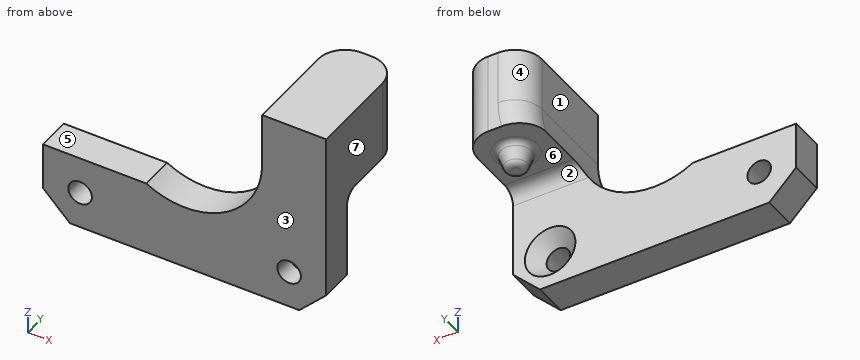
```python
from build123d import *

# Parameters (mm, degrees)
CROQUIS1_R              = 1.75
SALIENTE_EXTRUIR1_DEPTH = 5
CHAFL_N1_SIZE           = 2
SALIENTE_EXTRUIR2_DEPTH = 17.5
CROQUIS4_R              = 2.5
SALIENTE_EXTRUIR3_DEPTH = 3
NGULO_DE_SALIDA1_ANGLE  = 20
REDONDEO1_R             = 1
CHAFL_N2_SIZE           = 4
REDONDEO2_R             = 2
REDONDEO4_R             = 4


with BuildPart() as part:
    # Croquis1 → Saliente-Extruir1 (new body)
    with BuildSketch(Plane(origin=(0, 0, 0), x_dir=(1, 0, 0), z_dir=(0, 1, 0))):
        with BuildLine():
            Line((-21, 21), (21, 21))
            Line((21, 21), (21, -8))
            Line((21, -8), (11.5, -8))
            Line((11.5, -8), (11.5, 0))
            ThreePointArc((11.5, 0), (5.785436631, 9.938748562), (-5.678908346, 10))
            Line((-5.678908346, 10), (-21, 10))
            Line((-21, 10), (-21, 21))
        make_face()
        with Locations((-15.5, 15.5)):
            Circle(CROQUIS1_R, mode=Mode.SUBTRACT)
        with Locations((15.5, 15.5)):
            Circle(CROQUIS1_R, mode=Mode.SUBTRACT)
    extrude(amount=SALIENTE_EXTRUIR1_DEPTH)

    # Chaflán1
    chafl_n1_edges = [part.edges().sort_by_distance(p)[0] for p in [
        (13.75, 5, -15.5),
    ]]
    chamfer(chafl_n1_edges, length=CHAFL_N1_SIZE)

    # Croquis3 → Saliente-Extruir2 (add)
    with BuildSketch(Plane.XZ):
        with BuildLine():
            Line((10.781929326, -4), (21, -4))
            Line((21, -4), (21, 0))
            Line((21, 0), (21, 8))
            Line((21, 8), (11.5, 8))
            Line((11.5, 8), (11.5, 0))
            ThreePointArc((11.5, 0), (11.319058867, -2.031971056), (10.781929326, -4))
        make_face()
    extrude(amount=-SALIENTE_EXTRUIR2_DEPTH)

    # Croquis4 → Saliente-Extruir3 (add)
    with BuildSketch(Plane(origin=(0, 0, -4), x_dir=(-1, 0, 0), z_dir=(0, 0, -1))):
        with Locations((-16.25, 12)):
            Circle(CROQUIS4_R)
    extrude(amount=SALIENTE_EXTRUIR3_DEPTH)

    # Ángulo de salida1
    ngulo_de_salida1_faces = [part.faces().sort_by_distance(p)[0] for p in [
        (18.75, 12, -5.5),
    ]]
    draft(ngulo_de_salida1_faces, Plane(origin=(10.781929326, 17.5, -4), x_dir=(-1, 0, 0), z_dir=(0, 0, -1)), NGULO_DE_SALIDA1_ANGLE)

    # Redondeo1
    redondeo1_edges = [part.edges().sort_by_distance(p)[0] for p in [
        (18.75, 12, -4),
        (17.658089297, 12, -7),
    ]]
    fillet(redondeo1_edges, radius=REDONDEO1_R)

    # Chaflán2
    chafl_n2_edges = [part.edges().sort_by_distance(p)[0] for p in [
        (-21, 2.5, -21),
        (21, 2.5, -21),
    ]]
    chamfer(chafl_n2_edges, length=CHAFL_N2_SIZE)

    # Redondeo2
    redondeo2_edges = [part.edges().sort_by_distance(p)[0] for p in [
        (15.890964663, 5, -4),
    ]]
    fillet(redondeo2_edges, radius=REDONDEO2_R)

    # Redondeo4
    redondeo4_edges = [part.edges().sort_by_distance(p)[0] for p in [
        (21, 17.5, 2),
        (11.319058867, 17.5, -2.031971056),
        (11.5, 17.5, 4),
    ]]
    fillet(redondeo4_edges, radius=REDONDEO4_R)


solid = part.part
```
Can you work these out from the model? Positions are in its coordinate system, mm. Face numbers are marked on the shaded views. A direction names the side the tool comes from. Coordinates: 2 decimals unless noted, no trailing zeros. Loops run counter-clockwise (first coordinate to the right, second up) from the corner with the lowest first, then second, coordinate; pieces in that order, holes last. Notation, with made-up numbers: M 60,-5 L 118,-5 A27 cw 118,26 Z; hole C 81,58.25 d5. An arc over 180 degrees is marked long. Put each result on its own line as item: value. Start each with the question number.
(1) Which directions (+Z, -Z, +X, -X, +Y, -Y) give clear straight access to the entire face, cutting with the end or side of a thin tool? Please do the marked faces 4, 5, 6 and 7.
(2) Imagine slicing it at D-D on z = 5.5. List the corners of the cut face in (x, y) for me, and give its area (3 significant figures).
(3) Will these pins go through, and if not, where does the flat tip stop? pin 1 Ø3 at (x, z) = (-15.5, -15.5) entering from +Y; pin 2 Ø1.1 at (x, y) = (16.5, 12) entering from -Z; pin 3 Ø12 at (x, z) = (8, -15) entering from +Y; pin 4 Ø6 at (x, y) = (-5, 2) entering from +Z.
(4) I need wall thicknesses on probe 1 along X at (y, z) = (2.1, -15.5); probe 2 along Z at (x, y) = (15.5, 1.55); probe 3 along Z at (x, y) = (-15.5, 3). Which ranges of each line are inside material? Lowest first, please.
(5) Imagine slicing it at A-A on z = -15.5. List the corners of the cut face in (x, y) for me, and give its area (3 significant figures).
(6) We'd pull the mould along Y, two halves only. Please class the marked faces 1, 2 and 3: +Y half, -Y half, draft (parallel to the pull), parting line (faces both ways), or undercut.
(7) Imagine slicing it at C-C on y = 7.5. List the corners of the cut face in (x, z) for me, and give its area (3 significant figures).
(8) Imagine slicing it at B-B on y = 1.25. List the corners of the cut face in (x, z) for me, and give its area (3 significant figures).
Worked answers:
1. face 4: +Z, -X, +Y
1. face 5: +Z, -X, +Y, -Y
1. face 6: -Z
1. face 7: +Z, -Z, +X, +Y, -Y
2. outline: M 11.5,0 L 21,0 L 21,13.5 A4 ccw 17,17.5 L 15.5,17.5 A4 ccw 11.5,13.5 Z
2. area: 159 mm2
3. pin 1: passes through
3. pin 2: stops at z = -7
3. pin 3: stops at y = 5
3. pin 4: stops at z = -10
4. probe 1: x = -21 to -17.25, -13.75 to 13.75, 17.25 to 21
4. probe 2: z = -21 to -17.25, -13.75 to 8
4. probe 3: z = -21 to -17.25, -13.75 to -10
5. outline: M -21,0 L -17.25,0 L -17.25,5 L -21,5 Z; M -13.75,0 L 13.75,0 L 13.75,3 L 11.75,5 L -13.75,5 Z; M 17.25,0 L 21,0 L 21,5 L 19.25,5 L 17.25,3 Z
5. area: 171 mm2
6. face 1: draft
6. face 2: undercut
6. face 3: -Y half
7. outline: M 10.78,-4 L 21,-4 L 21,8 L 11.5,8 L 11.5,0 A11.5 cw Z
7. area: 115 mm2
8. outline: M -21,-17 L -17,-21 L 17,-21 L 21,-17 L 21,8 L 11.5,8 L 11.5,0 A11.5 cw -5.68,-10 L -21,-10 Z; hole C -15.5,-15.5 d3.5; hole C 15.5,-15.5 d3.5
8. area: 603 mm2
